Geometry check sheet. Reference: the model listing, model coordinates, mm. A direction names the side the tool comes from. Give positions to 0.01 mm unless a question says otherwise; leave off trailing zeros. Write each loop counter-clockwise with the first axis right and the second up, starting at its lowest first coordinate (ties: lowest second). Pieces come first, ordered by that corner, then holes. Notation, with made-up numbers: M 18.25,-21 L 67.25,-21 A29 cw 67.25,4 Z; hole C 45,-6 d11. An arc over 180 degrees is marked long. Use one line per item in the form item = value. Start each with the question number.
```python
from build123d import *

# Parameters (mm, degrees)
SKETCH1_W           = 100
SKETCH1_H           = 35
BOSS_EXTRUDE1_DEPTH = 5.9
SKETCH2_R           = 2.5
CUT_EXTRUDE1_DEPTH  = 10
FILLET1_R           = 10
SKETCH4_W           = 10
SKETCH4_H           = 3.45
CUT_EXTRUDE3_DEPTH  = 10
CUT_EXTRUDE5_REACH  = 7.9
SKETCH5_R           = 2.15
CUT_EXTRUDE6_REACH  = 7.9
SKETCH6_R           = 2.05


with BuildPart() as part:
    # Sketch1 → Boss-Extrude1 (new body)
    with BuildSketch(Plane(origin=(0, 0, 0), x_dir=(1, 0, 0), z_dir=(0, 1, 0))):
        Rectangle(SKETCH1_W, SKETCH1_H)
    extrude(amount=BOSS_EXTRUDE1_DEPTH)

    # Sketch2 → Cut-Extrude1 (cut)
    with BuildSketch(Plane(origin=(0, 5.9, 0), x_dir=(1, 0, 0), z_dir=(0, 1, 0))):
        with Locations((30, 0)):
            Circle(SKETCH2_R)
    extrude(amount=-CUT_EXTRUDE1_DEPTH, mode=Mode.SUBTRACT)

    # Fillet1
    fillet1_edges = [part.edges().sort_by_distance(p)[0] for p in [
        (50, 2.95, 17.5),
        (-50, 2.95, 17.5),
        (-50, 2.95, -17.5),
        (50, 2.95, -17.5),
    ]]
    fillet(fillet1_edges, radius=FILLET1_R)

    # Sketch4 → Cut-Extrude3 (cut)
    with BuildSketch(Plane(origin=(0, 5.9, 0), x_dir=(1, 0, 0), z_dir=(0, 1, 0))):
        with Locations((-35, 15.775)):
            Rectangle(SKETCH4_W, SKETCH4_H)
        with Locations((-35, -15.775)):
            Rectangle(SKETCH4_W, SKETCH4_H)
    extrude(amount=-CUT_EXTRUDE3_DEPTH, mode=Mode.SUBTRACT)

    # Sketch5 → Cut-Extrude5 (cut, up to next)
    with BuildSketch(Plane(origin=(0, 5.9, 0), x_dir=(1, 0, 0), z_dir=(0, 1, 0)), mode=Mode.PRIVATE) as cut_extrude5_sk1:
        with Locations((-5.3, 0)):
            Circle(SKETCH5_R)
    cut_extrude5_tool1 = extrude(cut_extrude5_sk1.sketch, amount=-CUT_EXTRUDE5_REACH, mode=Mode.PRIVATE) & part.part
    add(cut_extrude5_tool1.solids().sort_by_distance((-5.3, 5.9, 0))[0], mode=Mode.SUBTRACT)

    # Sketch6 → Cut-Extrude6 (cut, up to next)
    with BuildSketch(Plane(origin=(0, 5.9, 0), x_dir=(1, 0, 0), z_dir=(0, 1, 0)), mode=Mode.PRIVATE) as cut_extrude6_sk1:
        with Locations((-40, 14.05)):
            Circle(SKETCH6_R)
    cut_extrude6_tool1 = extrude(cut_extrude6_sk1.sketch, amount=-CUT_EXTRUDE6_REACH, mode=Mode.PRIVATE) & part.part
    add(cut_extrude6_tool1.solids().sort_by_distance((-40, 5.9, -14.05))[0], mode=Mode.SUBTRACT)
    # Sketch6 → Cut-Extrude6 (cut, up to next)
    with BuildSketch(Plane(origin=(0, 5.9, 0), x_dir=(1, 0, 0), z_dir=(0, 1, 0)), mode=Mode.PRIVATE) as cut_extrude6_sk2:
        with Locations((-30, 14.05)):
            Circle(SKETCH6_R)
    cut_extrude6_tool2 = extrude(cut_extrude6_sk2.sketch, amount=-CUT_EXTRUDE6_REACH, mode=Mode.PRIVATE) & part.part
    add(cut_extrude6_tool2.solids().sort_by_distance((-30, 5.9, -14.05))[0], mode=Mode.SUBTRACT)
    # Sketch6 → Cut-Extrude6 (cut, up to next)
    with BuildSketch(Plane(origin=(0, 5.9, 0), x_dir=(1, 0, 0), z_dir=(0, 1, 0)), mode=Mode.PRIVATE) as cut_extrude6_sk3:
        with Locations((-30, -14.05)):
            Circle(SKETCH6_R)
    cut_extrude6_tool3 = extrude(cut_extrude6_sk3.sketch, amount=-CUT_EXTRUDE6_REACH, mode=Mode.PRIVATE) & part.part
    add(cut_extrude6_tool3.solids().sort_by_distance((-30, 5.9, 14.05))[0], mode=Mode.SUBTRACT)
    # Sketch6 → Cut-Extrude6 (cut, up to next)
    with BuildSketch(Plane(origin=(0, 5.9, 0), x_dir=(1, 0, 0), z_dir=(0, 1, 0)), mode=Mode.PRIVATE) as cut_extrude6_sk4:
        with Locations((-40, -14.05)):
            Circle(SKETCH6_R)
    cut_extrude6_tool4 = extrude(cut_extrude6_sk4.sketch, amount=-CUT_EXTRUDE6_REACH, mode=Mode.PRIVATE) & part.part
    add(cut_extrude6_tool4.solids().sort_by_distance((-40, 5.9, 14.05))[0], mode=Mode.SUBTRACT)


solid = part.part
```
(1) Sectioned sample at B-B, the plane x = 30. Record the boundary of the cut face in (y, z).
(2) Thickness scan on probe 1 along X at (y, z) = (3.8, 0); probe 2 along Z at (x, y) = (-5.3, 4.1); probe 3 along Z at (x, y) = (30, 4.15). Record the ranges inside material, lowest first. Write a range as [from, to].
(3) Sectioned sample at A-A, the plane y = 4.2. Record the boundary of the cut face in (x, z).
(4) Draft check along X on faces 4 (the flat face through (5, 3, 17.5)), 5 (the cylindrical face through (46.99, 2.99, 14.65)), 6 (the cylindrical face through (-47.15, 2.99, 14.49)), 7 (the cylindrical face through (-28.6, 2.99, -12.55)). Enter one of: released by +X, released by -X, zero draft, split by the parting line, or undercut.
(5) Depth check by flat-ended pin: pin 1 (0.7 mm diameter, centred on y = 2.5, z = 16.5, fed in from -X); pin 2 (0.7 mm diameter, centred on y = 2, z = -17, fed in from +X); pin 3 (3.5 mm diameter, centred on x = -5.3, z = 0, fed in from +Y); pin 4 (1.1 mm diameter, centred on y = 3, z = 17, fed in from +X). Enter the tip coordinate at first touch or a pass-through.
(6) Tool access check on faces 1 (the flat face through (-35, 3, 14.05)), 2 (the flat face through (-35, 3, -14.05)), 3 (the cylindrical face through (46.99, 2.99, -14.65)). Record the directions out of +Z, -Z, +X, -X, +Y, -Y that give a thin tool (end or side, any length) a straight path to the whole face; none if there is none.
Numbers:
q1.outline = M 0,-17.5 L 5.9,-17.5 L 5.9,-2.5 L 0,-2.5 Z; M 0,2.5 L 5.9,2.5 L 5.9,17.5 L 0,17.5 Z
q2.probe_1 = [-50, -7.45], [-3.15, 27.5], [32.5, 50]
q2.probe_2 = [-17.5, -2.15], [2.15, 17.5]
q2.probe_3 = [-17.5, -2.5], [2.5, 17.5]
q3.outline = M -50,-7.5 A10 ccw -40,-17.5 L -40,-16.1 A2.05 cw long -37.95,-14.05 L -32.05,-14.05 A2.05 cw long -30,-16.1 L -30,-17.5 L 40,-17.5 A10 ccw 50,-7.5 L 50,7.5 A10 ccw 40,17.5 L -30,17.5 L -30,16.1 A2.05 cw long -32.05,14.05 L -37.95,14.05 A2.05 cw long -40,16.1 L -40,17.5 A10 ccw -50,7.5 Z; hole C -5.3,0 d4.3; hole C 30,0 d5
q4.face_4 = zero draft
q4.face_5 = released by +X
q4.face_6 = released by -X
q4.face_7 = undercut
q5.pin_1 = -45.02
q5.pin_2 = 44.03
q5.pin_3 = through
q5.pin_4 = 44.46
q6.face_1 = +Z, +Y, -Y
q6.face_2 = -Z, +Y, -Y
q6.face_3 = -Z, +X, +Y, -Y
